Can you work these out from the model? Positions are in its coordinate system, mm. Face numbers are marked on the shaded views. Give positions to 0.01 mm unless a question says otherwise; leave off trailing zeros. Write each loop counter-clockwise with the first axis right and the second up, starting at its lowest first coordinate (ties: lowest second). Pieces come first, ordered by that corner, then holes. Notation, with made-up numbers: (-21, 40.25) -> (34, 40.25) arc R16 cw to (34, 46.25) -> close; hole circle Ø3 at (-39, -12). An arc over 180 degrees is marked (long way). Answer as CSV lines item,"result". Start each with the question number.
1. If we section it at C-C on y = 5.65: Write out the boundary of the cut face in (x, z), plus the area to 3 significant figures.
2. If we section it at D-D on x = -8.5: Write out the boundary of the cut face in (y, z), plus the area to 3 significant figures.
3. I need wall thicknesses on line 1 (Y direction, x = 0, z = -6.5); line 2 (Z direction, x = -5, y = 3.7); line 3 (X direction, y = 4.3, z = -4.5). Which ranges of each line are inside material? Lowest first, please. Write a range as [from, to].
4. If we mould it in two halves opening along X, with no side actions, what happens to the marked faces 1, 2 and 3? For each: pulls with the +X half, pulls with the -X half, needs draft (parallel to the pull), parting line crosses it, or undercut.
5. I'm going to push flat-ended pins straight in: P1, Ø5.5, axis at x = 1.5, z = -1, coming from the +Y side; P2, Ø2, axis at y = 5.5, z = -5, coming from the -X side; P3, Ø1.6, axis at y = 5.5, z = -12.5, coming from the +X side. Where does each tip first touch, or does it pass through?
6. If we section it at A-A on z = -8: Write out the boundary of the cut face in (x, y), plus the area to 3 significant figures.
Autodesk Inventor part; units mm, degrees
ref_plane "YZ Plane" through (0, 0, 0) normal (1, 0, 0) x (0, 1, 0)
ref_plane "XZ Plane" through (0, 0, 0) normal (0, 1, 0) x (-1, 0, 0)
ref_plane "XY Plane" through (0, 0, 0) normal (0, 0, 1) x (1, 0, 0)
sketch "Skizze1" plane through (0, 0, 0) normal (0, 1, 0) x (-1, 0, 0)
  line L0 (10, 12.5) -> (-10, 12.5)
  line L1 (-10, 12.5) -> (-10, -12.5)
  line L2 (-10, -12.5) -> (10, -12.5)
  line L3 (10, -12.5) -> (10, 12.5)
  line L4 (10, 12.5) -> (-10, -12.5) construction
  line L5 (-10, 12.5) -> (10, -12.5) construction
  point P0 (0, 0)
  dimension "d0" = 20
  dimension "d1" = 25
extrude "Extrusion1" add sketch "Skizze1" along normal blind 5
fillet "Rundung1" radius 1 4 edges at (-10, 5, 0) (-10, 0, 0) (10, 5, 0) (10, 0, 0)
sketch "Skizze2" plane through (9, 0, -12.5) normal (0, 0, -1) x (-1, 0, 0)
  line L0 (0, 5) -> (18, 5)
  line L1 (6, 4) -> (12, 4)
  line L2 (12, 4) -> (12, 6)
  line L3 (12, 6) -> (6, 6)
  line L4 (6, 6) -> (6, 4)
  line L5 (6, 4) -> (12, 6) construction
  line L6 (12, 4) -> (6, 6) construction
  point P0 (9, 0)
  point P1 (9, 5)
  dimension "d5" = 2
  dimension "d6" = 6
extrude "Extrusion2" add sketch "Skizze2" along normal blind 3 and the other way blind 1.5
chamfer "Fasen1" distance 1 angle 45 1 edges at (0, 5, -11)
chamfer "Fasen2" distance 1 angle 45 2 edges at (-3, 5, -10.5002) (-3, 5, -11.75)
chamfer "Fasen3" distance 1 angle 45 2 edges at (3, 5, -10.5003) (3, 5, -11.75)
fillet "Rundung2" radius 1 5 edges at (3, 5.4998, -12.5) (3, 4.5, -12.5) (0, 4, -12.5) (-3, 4.5, -12.5) (-3, 5.4998, -12.5)
properties part number "Batterie" material "Nylon 6/6"
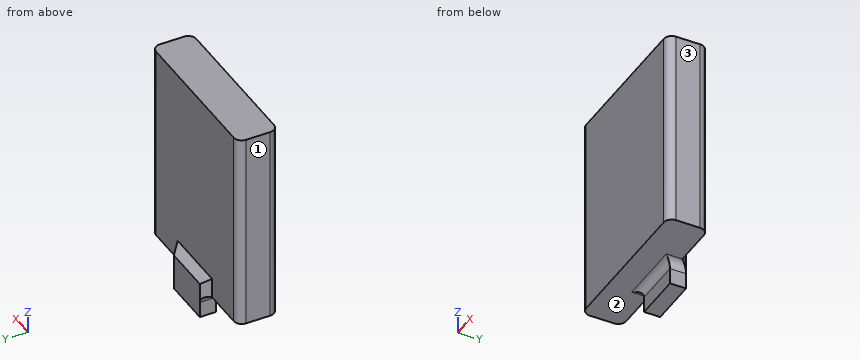
Computed values:
1,outline,"(-3.35, -12.74) arc R1 cw to (-3, -13.5) -> (-3, -15.5) -> (3, -15.5) -> (3, -13.5) arc R1 cw to (3.35, -12.74) -> (3.35, -10.65) -> (-3.35, -10.65) -> close"
1,area,"30.7 mm2"
2,outline,"(0, -12.5) -> (5, -12.5) -> (5, 12.5) -> (0, 12.5) -> close"
2,area,"125 mm2"
3,line 1,"y = [0, 5]"
3,line 2,"z = [-12.5, 12.5]"
3,line 3,"x = [-9.95, 9.95]"
4,face 1,"pulls with the -X half"
4,face 2,"needs draft"
4,face 3,"pulls with the +X half"
5,P1,"stops at y = 5"
5,P2,"stops at x = -9.87"
5,P3,"stops at x = 9.71"
6,outline,"(-10, 1) arc R1 ccw to (-9, 0) -> (9, 0) arc R1 ccw to (10, 1) -> (10, 4) arc R1 ccw to (9, 5) -> (-9, 5) arc R1 ccw to (-10, 4) -> close"
6,area,"99.1 mm2"
